Work out the finished part from the listing and answer in its coordinate system (mm). Face numbers are marked on the shaded views. A direction names the side the tool comes from. Round coordinates to 2 decimals unless told otherwise and drop trailing zeros. Loops run counter-clockwise (first coordinate to the right, second up) from the corner with the lowest first, then second, coordinate; pieces in that order, holes last. Notation, with made-up numbers: M 60.25,21 L 104.25,21 A25 ccw 104.25,37 Z; hole C -15,-16.5 d5. An arc over 180 degrees is marked long. One line per item, written item: value.
```python
from build123d import *

# Parameters (mm, degrees)
SKETCH1_W           = 125
SKETCH1_H           = 90
SKETCH1_W_2         = 120
SKETCH1_H_2         = 85
BOSS_EXTRUDE1_DEPTH = 2.5
SKETCH1_3_W         = 125
SKETCH1_3_H         = 90
SKETCH1_3_W_2       = 120
SKETCH1_3_H_2       = 85
BOSS_EXTRUDE2_DEPTH = 93
SKETCH2_W           = 32
SKETCH2_H           = 36
CUT_EXTRUDE1_DEPTH  = 5
CUT_EXTRUDE2_DEPTH  = 10
SKETCH6_W           = 8
SKETCH6_H           = 8
CUT_EXTRUDE3_DEPTH  = 10
SKETCH7_W           = 20
SKETCH7_H           = 10
CUT_EXTRUDE4_DEPTH  = 10


with BuildPart() as part:
    # Sketch1 → Boss-Extrude1 (new body)
    # profile 1 of 2: a face of its own
    with BuildSketch(Plane(origin=(0, 0, 0), x_dir=(1, 0, 0), z_dir=(0, 1, 0))):
        Rectangle(SKETCH1_W, SKETCH1_H)
        Rectangle(SKETCH1_W_2, SKETCH1_H_2, mode=Mode.SUBTRACT)
    # profile 2 of 2: a face of its own
    with BuildSketch(Plane(origin=(0, 0, 0), x_dir=(1, 0, 0), z_dir=(0, 1, 0))):
        Rectangle(SKETCH1_W_2, SKETCH1_H_2)
    extrude(amount=BOSS_EXTRUDE1_DEPTH)

    # Sketch1_3 → Boss-Extrude2 (add)
    with BuildSketch(Plane(origin=(0, 0, 0), x_dir=(1, 0, 0), z_dir=(0, 1, 0))):
        Rectangle(SKETCH1_3_W, SKETCH1_3_H)
        Rectangle(SKETCH1_3_W_2, SKETCH1_3_H_2, mode=Mode.SUBTRACT)
    extrude(amount=BOSS_EXTRUDE2_DEPTH)

    # Sketch2 → Cut-Extrude1 (cut)
    with BuildSketch(Plane(origin=(62.5, 0, 0), x_dir=(0, 0, -1), z_dir=(1, 0, 0))):
        with Locations((-22.5, 58)):
            Rectangle(SKETCH2_W, SKETCH2_H)
        with BuildLine():
            Line((-23, 81.625), (-22, 81.625))
            ThreePointArc((-22, 81.625), (-20.875, 80.5), (-22, 79.375))
            Line((-22, 79.375), (-23, 79.375))
            ThreePointArc((-23, 79.375), (-24.125, 80.5), (-23, 81.625))
        make_face()
        with BuildLine():
            Line((-23, 34.375), (-22, 34.375))
            ThreePointArc((-22, 34.375), (-20.875, 35.5), (-22, 36.625))
            Line((-22, 36.625), (-23, 36.625))
            ThreePointArc((-23, 36.625), (-24.125, 35.5), (-23, 34.375))
        make_face()
    extrude(amount=-CUT_EXTRUDE1_DEPTH, mode=Mode.SUBTRACT)

    # Sketch5 → Cut-Extrude2 (cut)
    with BuildSketch(Plane.XY.offset(45)):
        with BuildLine():
            Line((-37.5, 10.5), (-37.5, 12.5))
            ThreePointArc((-37.5, 12.5), (-34.5, 15.5), (-31.5, 12.5))
            Line((-31.5, 12.5), (-31.5, 10.5))
            ThreePointArc((-31.5, 10.5), (-34.5, 7.5), (-37.5, 10.5))
        make_face()
        with BuildLine():
            Line((-21.5, 10.5), (-21.5, 12.5))
            ThreePointArc((-21.5, 12.5), (-18.5, 15.5), (-15.5, 12.5))
            Line((-15.5, 12.5), (-15.5, 10.5))
            ThreePointArc((-15.5, 10.5), (-18.5, 7.5), (-21.5, 10.5))
        make_face()
        with BuildLine():
            Line((-5.5, 10.5), (-5.5, 12.5))
            ThreePointArc((-5.5, 12.5), (-2.5, 15.5), (0.5, 12.5))
            Line((0.5, 12.5), (0.5, 10.5))
            ThreePointArc((0.5, 10.5), (-2.5, 7.5), (-5.5, 10.5))
        make_face()
    extrude(amount=-CUT_EXTRUDE2_DEPTH, mode=Mode.SUBTRACT)

    # Sketch6 → Cut-Extrude3 (cut)
    with BuildSketch(Plane(origin=(62.5, 0, 0), x_dir=(0, 0, -1), z_dir=(1, 0, 0))):
        with Locations((15, 55)):
            Rectangle(SKETCH6_W, SKETCH6_H)
    extrude(amount=-CUT_EXTRUDE3_DEPTH, mode=Mode.SUBTRACT)

    # Sketch7 → Cut-Extrude4 (cut)
    with BuildSketch(Plane(origin=(0, 0, -45), x_dir=(-1, 0, 0), z_dir=(0, 0, -1))):
        with Locations((-22.5, 65)):
            Rectangle(SKETCH7_W, SKETCH7_H)
        with Locations((2.5, 65)):
            Rectangle(SKETCH7_W, SKETCH7_H)
    extrude(amount=-CUT_EXTRUDE4_DEPTH, mode=Mode.SUBTRACT)


solid = part.part
```
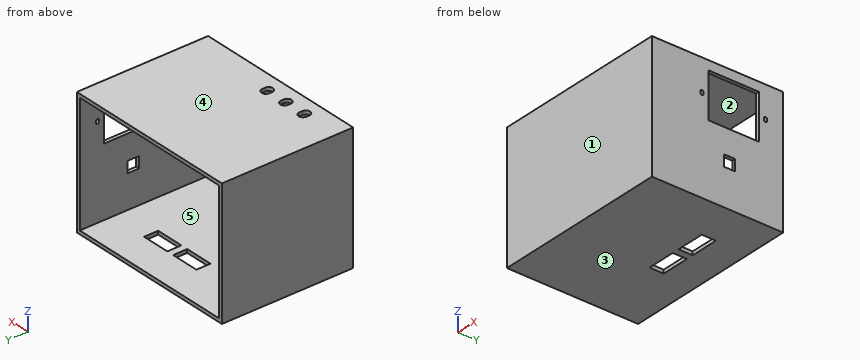
1) Find the intervals of material crossed by probe 1 along X at (y, z) = (39.5, 38); probe 2 along Z at (x, y) = (2.5, 82.5); probe 3 along Y at (x, z) = (-57, -19.5), in increasing order. Write a range as from..to.
Check values:
probe 1: -62.5..-60, 60..62.5
probe 2: -45..-42.5, 42.5..45
probe 3: 0..2.5
2) For the marked faces 4 and 5, determine the directions among +Z, -Z, +X, -X, +Y, -Y from which every point of the face is accessible in a straight line to the end or side of a thin tool.
Check values:
face 4: +Z, +X, -X, +Y, -Y
face 5: +Y
3) Each of these flat-tipped pins is pushed along its axis until it touches: pin 1 (8 mm diameter, centred on x = -2, z = -7.5, fed in from +Y); pin 2 (4 mm diameter, centred on y = 64, z = 21, fed in from +X). Where does it stop, or does it pass through?
Check values:
pin 1: y = 2.5
pin 2: x = -60
4) Find section C-C (z = 8). Give the vertices of the cut face in (x, y), then the cut area to 3 significant figures.
Check values:
outline: M -62.5,0 L 62.5,0 L 62.5,40 L 60,40 L 60,2.5 L -60,2.5 L -60,93 L -62.5,93 Z; M 60,76 L 62.5,76 L 62.5,93 L 60,93 Z
area: 675 mm2
5) The mould has two halves that part along Z. Classify the marked faces 1, 2 and 3: +Z half, -Z half, draft (parallel to the pull), parting line (faces both ways), or undercut.
Check values:
face 1: draft
face 2: undercut
face 3: -Z half
6) Find section A-A (y = 67). Give the vertices of the cut face in (x, z), then the cut area to 3 significant figures.
Check values:
outline: M -62.5,-45 L -12.5,-45 L -12.5,-42.5 L -60,-42.5 L -60,42.5 L 60,42.5 L 60,38.5 L 62.5,38.5 L 62.5,45 L -62.5,45 Z; M 7.5,-45 L 12.5,-45 L 12.5,-42.5 L 7.5,-42.5 Z; M 32.5,-45 L 62.5,-45 L 62.5,6.5 L 60,6.5 L 60,-42.5 L 32.5,-42.5 Z
area: 870 mm2
7) Find section D-D (x = -34.5). Give the vertices of the cut face in (y, z), then the cut area to 4 significant figures.
Check values:
outline: M 0,-45 L 93,-45 L 93,-42.5 L 2.5,-42.5 L 2.5,42.5 L 7.5,42.5 L 7.5,45 L 0,45 Z; M 15.5,42.5 L 93,42.5 L 93,45 L 15.5,45 Z
area: 657.5 mm2
8) Find section B-B (x = -2.5). Give the vertices of the cut face in (y, z).
Check values:
outline: M 0,-45 L 60,-45 L 60,-42.5 L 2.5,-42.5 L 2.5,42.5 L 7.5,42.5 L 7.5,45 L 0,45 Z; M 15.5,42.5 L 93,42.5 L 93,45 L 15.5,45 Z; M 70,-45 L 93,-45 L 93,-42.5 L 70,-42.5 Z
